from build123d import *

# Parameters (mm, degrees)
BOSS_EXTRUDE1_DEPTH     = 75
BOSS_EXTRUDE2_DEPTH     = 75
SKETCH6_W               = 32
SKETCH6_H               = 32
CUT_EXTRUDE1_DEPTH      = 232.532584422
FILLET1_START           = -75
FILLET1_DEPTH           = 150
FILLET1_START_2         = -40.56574
FILLET1_2_DEPTH         = 24.56574
FILLET1_START_3         = 16
FILLET1_3_DEPTH         = 10
FILLET1_START_4         = -26
FILLET1_4_DEPTH         = 101
FILLET1_5_DEPTH         = 34.43426
FILLET1_START_5         = -113.13708499
FILLET1_6_OUTLINE_W     = 32
FILLET1_6_OUTLINE_H     = 32
FILLET1_6_DEPTH         = 29.279073903
CUT_EXTRUDE3_DEPTH      = 232.532584422
CUT_EXTRUDE3_DEPTH_BACK = 232.532584422
SKETCH10_W              = 110
SKETCH10_H              = 254.558441228
CUT_EXTRUDE4_DEPTH      = 232.532584422
CUT_EXTRUDE4_DEPTH_BACK = 232.532584422
SKETCH11_R              = 5
SKETCH11_R_2            = 3
FILLET2_R               = 15


with BuildPart() as part:
    # Sketch3 → Boss-Extrude1 (new, symmetric)
    with BuildSketch(Plane(origin=(0, 0, 0), x_dir=(0, 0, -1), z_dir=(1, 0, 0))):
        with BuildLine():
            Line((7.071067812, -7.071067812), (141.421356237, 127.279220614))
            Line((141.421356237, 127.279220614), (141.421356237, 167.279220614))
            Line((141.421356237, 167.279220614), (113.13708499, 167.279220614))
            Line((113.13708499, 167.279220614), (113.13708499, 127.279220614))
            Line((113.13708499, 127.279220614), (-7.071067812, 7.071067812))
            ThreePointArc((-7.071067812, 7.071067812), (-7.071067812, -7.071067812), (7.071067812, -7.071067812))
        make_face()
    extrude(amount=BOSS_EXTRUDE1_DEPTH, both=True)

    # Sketch9 → Boss-Extrude2 (add, symmetric)
    with BuildSketch(Plane(origin=(0, 0, 0), x_dir=(0, 0, -1), z_dir=(1, 0, 0))):
        Polygon((57.175144213, 127.279220614), (57.175144213, 167.279220614), (77.175144213, 167.279220614), (77.175144213, 127.279220614), (77.175144213, 91.317279836), (57.175144213, 71.317279836), align=None)
    extrude(amount=BOSS_EXTRUDE2_DEPTH, both=True)

    # Sketch6 → Cut-Extrude1 (cut, through all)
    with BuildSketch(Plane.XY):
        with Locations((0, 147.279220614)):
            Rectangle(SKETCH6_W, SKETCH6_H)
        Polygon((-26, 167.279220614), (-75, 142.279220614), (-75, 167.279220614), align=None)
        Polygon((26, 167.279220614), (75, 167.279220614), (75, 142.279220614), align=None)
    extrude(amount=-CUT_EXTRUDE1_DEPTH, mode=Mode.SUBTRACT)

    # Fillet1: read off the stored shape, not the designer's step
    # Fillet1 outline → Fillet1 (add)
    with BuildSketch(Plane.YZ.offset(FILLET1_START)):
        with BuildLine():
            Line((131.279220614, -113.13708499), (131.279220614, -105.877452163))
            ThreePointArc((131.279220614, -105.877452163), (113.530191873, -96.544561619), (98.00014671, -83.858011087))
            Line((98.00014671, -83.858011087), (127.279220614, -113.13708499))
            Line((127.279220614, -113.13708499), (131.279220614, -113.13708499))
        make_face()
        with BuildLine():
            Line((71.317279836, -57.175144213), (112.738636074, -57.175144213))
            ThreePointArc((112.738636074, -57.175144213), (74.470292837, -49.563097464), (42.027957955, -27.885822331))
            Line((42.027957955, -27.885822331), (71.317279836, -57.175144213))
        make_face()
    extrude(amount=FILLET1_DEPTH)

    # Fillet1 2 outline → Fillet1 2 (add)
    with BuildSketch(Plane.YZ.offset(FILLET1_START_2)):
        with BuildLine():
            ThreePointArc((167.279220614, -113.13708499), (148.943103424, -111.174049686), (131.279220614, -105.877452163))
            Line((131.279220614, -105.877452163), (131.279220614, -113.13708499))
            Line((131.279220614, -113.13708499), (167.279220614, -113.13708499))
        make_face()
    extrude(amount=FILLET1_2_DEPTH)

    # Fillet1 3 outline → Fillet1 3 (add)
    with BuildSketch(Plane.YZ.offset(FILLET1_START_3)):
        with BuildLine():
            ThreePointArc((167.279220614, -113.13708499), (148.943103424, -111.174049686), (131.279220614, -105.877452163))
            Line((131.279220614, -105.877452163), (131.279220614, -113.13708499))
            Line((131.279220614, -113.13708499), (167.279220614, -113.13708499))
        make_face()
    extrude(amount=FILLET1_3_DEPTH)

    # Fillet1 4 outline → Fillet1 4 (add)
    with BuildSketch(Plane.YZ.offset(FILLET1_START_4)):
        with BuildLine():
            Line((131.279220614, -113.13708499), (167.279220614, -113.13708499))
            ThreePointArc((167.279220614, -113.13708499), (148.943103424, -111.174049686), (131.279220614, -105.877452163))
            Line((131.279220614, -105.877452163), (131.279220614, -113.13708499))
        make_face()
    extrude(amount=FILLET1_4_DEPTH)

    # Fillet1 5 outline → Fillet1 5 (add)
    with BuildSketch(Plane.YZ.offset(FILLET1_START)):
        with BuildLine():
            Line((131.279220614, -113.13708499), (167.279220614, -113.13708499))
            ThreePointArc((167.279220614, -113.13708499), (148.943103424, -111.174049686), (131.279220614, -105.877452163))
            Line((131.279220614, -105.877452163), (131.279220614, -113.13708499))
        make_face()
    extrude(amount=FILLET1_5_DEPTH)

    # Fillet1 6 outline → Fillet1 6 (cut)
    with BuildSketch(Plane.XY.offset(FILLET1_START_5)):
        Polygon((75, 167.279220614), (26, 167.279220614), (75, 142.279220614), align=None)
        Polygon((-26, 167.279220614), (-75, 167.279220614), (-75, 142.279220614), align=None)
        with Locations((0, 147.279220614)):
            Rectangle(FILLET1_6_OUTLINE_W, FILLET1_6_OUTLINE_H)
    extrude(amount=FILLET1_6_DEPTH, mode=Mode.SUBTRACT)

    # Sketch10 → Cut-Extrude3 (cut, two sides: drawn at the far end of the back side and taken through both)
    with BuildSketch(Plane.XY.offset(-CUT_EXTRUDE3_DEPTH_BACK)):
        Rectangle(SKETCH10_W, SKETCH10_H)
    extrude(amount=CUT_EXTRUDE3_DEPTH + CUT_EXTRUDE3_DEPTH_BACK, mode=Mode.SUBTRACT)

    # Sketch11 → Cut-Extrude4 (cut, two sides: drawn at the far end of the back side and taken through both)
    with BuildSketch(Plane(origin=(0, 0, 0), x_dir=(0, 0, -1), z_dir=(1, 0, 0)).offset(-CUT_EXTRUDE4_DEPTH_BACK)):
        Circle(SKETCH11_R)
        with Locations((62.404851943, 114.904851943)):
            Circle(SKETCH11_R_2)
        with BuildLine():
            Line((118.793939239, 114.551298552), (115.258405333, 111.015764646))
            ThreePointArc((115.258405333, 111.015764646), (111.015764646, 111.015764646), (111.015764646, 115.258405333))
            Line((111.015764646, 115.258405333), (114.551298552, 118.793939239))
            ThreePointArc((114.551298552, 118.793939239), (118.793939239, 118.793939239), (118.793939239, 114.551298552))
        make_face()
    extrude(amount=CUT_EXTRUDE4_DEPTH + CUT_EXTRUDE4_DEPTH_BACK, mode=Mode.SUBTRACT)

    # Fillet2
    fillet2_edges = [part.edges().sort_by_distance(p)[0] for p in [
        (75, 142.279220614, -127.279220614),
        (75, 142.279220614, -67.175144213),
        (-75, 142.279220614, -127.279220614),
        (-75, 142.279220614, -67.175144213),
    ]]
    fillet(fillet2_edges, radius=FILLET2_R)


solid = part.part
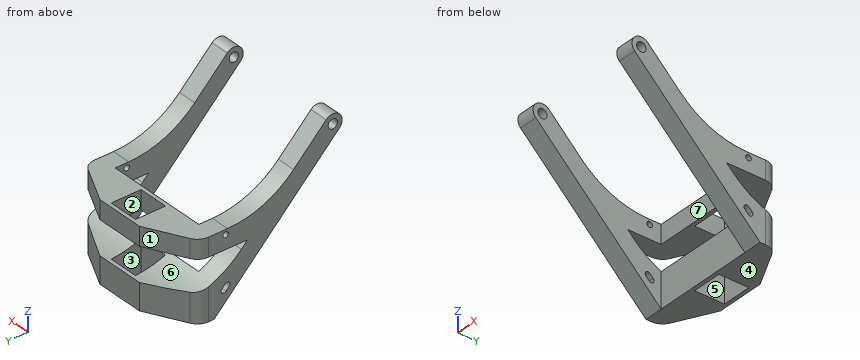
Part model, mm, in its own coordinate system. Face numbers are marked on the shaded views. A direction names the side the tool comes from. Coordinates: 2 decimals unless noted, no trailing zeros. Loops run counter-clockwise (first coordinate to the right, second up) from the corner with the lowest first, then second, coordinate; pieces in that order, holes last. Notation, with made-up numbers: M 67,-39 L 118,-39 A28 cw 118,-5 Z; hole C 50.5,22.25 d3. An arc over 180 degrees is marked long. Use a Markdown table: item, result. Add a question column.
Q1. Probe L1, parallel to Y at x = -0.5, z = -119; L2, parallel to X at y = 11.5, z = -6; L3, parallel to Z at x = -66, y = 0. List the from-to ranges inside material, lowest first.
Q2. Pin check, flat tips, straight feed: P1, Ø6, axis at y = 149.5, z = -62.5, coming from the +X side; P2, Ø12, axis at x = -36.5, z = -65.5, coming from the -Y side; P3, Ø16, axis at y = 145, z = -118.5, coming from the +X side; P4, Ø9, axis at y = 0, z = 0, coming from the -X side. Stop position of each tip, or through.
Q3. Which spindle directions (+Z, -Z, +X, -X, +Y, -Y) get a long thin tool onto all of the face, cutting with end or side? Do the marked faces 5, 6 and 7. Say none if no direction does.
Q4. Cut at A-A (x = 12). Write the cut outline in (y, z), and give its area (3 significant figures).
Q5. Cut at B-B (y = 14.5). Write the cut outline in (x, z).
Q6. Mould opens along Y. For the marked faces 1, 2, 3 and 4 say: +Y half, -Y half, draft (parallel to the pull), parting line (faces both ways), or undercut.
Q7. Cut at D-D (x = -64.5). Write the cut outline in (y, z), and give its area (3 significant figures).
Q8. Cut at C-C (z = 0). Write the cut outline in (x, y).
Worked out:
| question | item | result |
|---|---|---|
| 1 | L1 | y = 127.28 to 131.28, 163.28 to 167.28 |
| 1 | L2 | x = -75 to -55, 55 to 75 |
| 1 | L3 | z = -14.14 to -5, 5 to 10 |
| 2 | P1 | stops at x = 66.73 |
| 2 | P2 | stops at y = 127.28 |
| 2 | P3 | stops at x = 74.48 |
| 2 | P4 | passes through |
| 3 | face 5 | +Z, -Z |
| 3 | face 6 | +X, -X, +Y |
| 3 | face 7 | +Z, -Z, -Y |
| 4 | outline | M 127.28,-141.42 L 131.28,-141.42 L 131.28,-105.88 A100 cw 127.28,-104.16 Z; M 127.28,-77.18 L 131.28,-77.18 L 131.28,-57.18 L 127.28,-57.18 Z; M 163.28,-141.42 L 167.28,-141.42 L 167.28,-113.14 A100 cw 163.28,-113 Z; M 163.28,-77.18 L 167.28,-77.18 L 167.28,-57.18 L 163.28,-57.18 Z |
| 4 | area | 419 mm2 |
| 5 | outline | M -75,-28.64 L -55,-28.64 L -55,-0.36 L -75,-0.36 Z; M 55,-28.64 L 75,-28.64 L 75,-0.36 L 55,-0.36 Z |
| 6 | face 1 | +Y half |
| 6 | face 2 | undercut |
| 6 | face 3 | undercut |
| 6 | face 4 | draft |
| 7 | outline | M -7.07,-7.07 L 127.28,-141.42 L 147.64,-141.42 L 147.64,-110.9 A100 cw 98,-83.86 L 91.32,-77.18 L 147.64,-77.18 L 147.64,-57.18 L 112.74,-57.18 A100 cw 42.03,-27.89 L 7.07,7.07 A10 ccw Z; hole C 0,0 d10; hole M 111.02,-115.26 L 114.55,-118.79 A3 ccw 118.79,-114.55 L 115.26,-111.02 A3 ccw Z; hole C 114.9,-62.4 d6 |
| 7 | area | 5,910 mm2 |
| 8 | outline | M -75,-10 L -55,-10 L -55,-5 L -75,-5 Z; M -75,5 L -55,5 L -55,14.14 L -75,14.14 Z; M 55,-10 L 75,-10 L 75,-5 L 55,-5 Z; M 55,5 L 75,5 L 75,14.14 L 55,14.14 Z |
